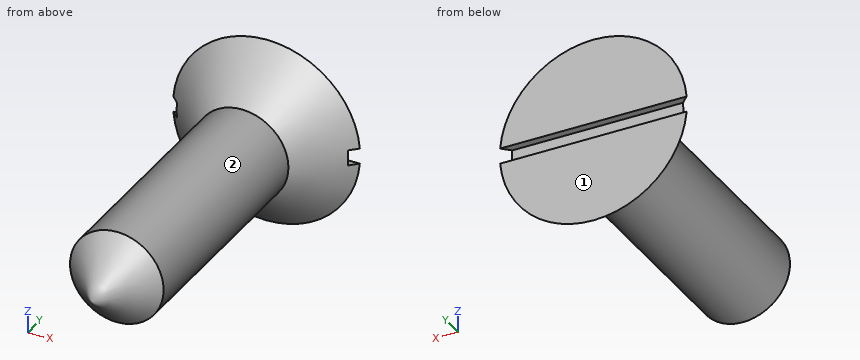
from build123d import *

# Parameters (mm, degrees)
SKETCH2_W          = 2
SKETCH2_H          = 2
CUT_EXTRUDE1_DEPTH = 50


with BuildPart() as part:
    # Sketch1 → Revolve2 (revolve)
    with BuildSketch(Plane.XY):
        Polygon((12, 12.4), (0, 12.4), (0, 6.48), (0, -29.6), (6, -23.6), (6, 6.4), align=None)
    revolve(axis=Axis((0, -39.28, 0), (0, 1, 0)))

    # Sketch2 → Cut-Extrude1 (cut, symmetric)
    with BuildSketch(Plane(origin=(0, 0, 0), x_dir=(0, 0, -1), z_dir=(1, 0, 0))):
        with Locations((0, 12.4)):
            Rectangle(SKETCH2_W, SKETCH2_H)
    extrude(amount=CUT_EXTRUDE1_DEPTH, both=True, mode=Mode.SUBTRACT)


solid = part.part
Input: part model. Units: mm. Frame: model coordinates. Face numbers are marked on the shaded views. A direction names the side the tool comes from. Coordinates: 2 decimals unless noted, no trailing zeros. Order: outer loops, then holes, each group sorted by start corner. A loop starts at its lowest first (then second) coordinate and runs counter-clockwise, first axis right, second up. Notation, with made-up numbers: M 1.5,79.25 L 34.5,79.25 A20 ccw 34.5,83.25 Z; hole C 41.5,65.25 d11. An arc over 180 degrees is marked long. Write item = value, one per line. Start each with the question number.
(1) Reachability of the marked faces 1 and 2 from +Z, -Z, +X, -X, +Y, -Y: full face, straight path, thin tool, end or side. Return the list, or none.
(2) Section A-A on y = 9.5. Output: boundary loops of the cut face in (x, z), and give its area (3 significant figures).
(3) Section B-B on y = -25.5. Output: boundary loops of the cut face in (x, z).
(4) Line query: line 1 along Z through (x, y) = (0, -19.5); line 2 along X through (y, z) = (-2.5, 2.25); line 3 along Y through (x, z) = (8.75, -0.5). Output: solid intervals per line, ascending. Write a range as [from, to].
(5) First-contact query: P1, Ø8, axis at x = -8.5, y = -5, coming from the +Z side; P2, Ø8, axis at x = 3, y = -10.5, coming from the -Z side; P3, Ø4, axis at x = -7.5, z = 9.5, coming from the -Y side. Flat tips, straight axial feed; report the tip coordinate or a pass-through.
Result set:
q1.face_1 = +Z, -Z, +X, -X, +Y
q1.face_2 = -Y
q2.outline = C 0,0 d18.2
q2.area = 260 mm²
q3.outline = C 0,0 d8.2
q4.line_1 = [-6, 6]
q4.line_2 = [-5.56, 5.56]
q4.line_3 = [9.16, 11.4]
q5.P1 = 3.97
q5.P2 = -6
q5.P3 = 10.5
